```python
from build123d import *

# Parameters (mm, degrees)
SKETCH1_R           = 15
BOSS_EXTRUDE1_DEPTH = 30
SKETCH8_W           = 30
SKETCH8_H           = 15
REVOLVE1_ANGLE      = 180
SKETCH9_W           = 30
SKETCH9_H           = 30
BOSS_EXTRUDE3_DEPTH = 15
SKETCH10_R          = 5
CUT_EXTRUDE1_DEPTH  = 30
SKETCH13_R          = 16
CUT_EXTRUDE2_DEPTH  = 10
SKETCH14_W          = 10
SKETCH14_H          = 15
CUT_EXTRUDE3_DEPTH  = 67
CUT_EXTRUDE4_START  = -7
SKETCH15_R          = 11
SKETCH15_R_2        = 5
CUT_EXTRUDE4_DEPTH  = 7
SKETCH16_R          = 11
SKETCH16_R_2        = 5
CUT_EXTRUDE5_DEPTH  = 7


with BuildPart() as part:
    # Sketch1 → Boss-Extrude1 (new body)
    with BuildSketch(Plane(origin=(0, 0, 0), x_dir=(1, 0, 0), z_dir=(0, 1, 0))):
        with Locations(Location((0, 0, 0), (0, 0, 270))):
            Circle(SKETCH1_R)
    extrude(amount=BOSS_EXTRUDE1_DEPTH)

    # Sketch8 → Revolve1 (revolve)
    with BuildSketch(Plane(origin=(0, 30, 0), x_dir=(1, 0, 0), z_dir=(0, 1, 0))):
        with Locations((0, -7.5)):
            Rectangle(SKETCH8_W, SKETCH8_H)
    revolve(axis=Axis((15, 30, 0), (-1, 0, 0)), revolution_arc=REVOLVE1_ANGLE)

    # Sketch9 → Boss-Extrude3 (add)
    with BuildSketch(Plane.XZ.offset(-30)):
        Rectangle(SKETCH9_W, SKETCH9_H)
    extrude(amount=BOSS_EXTRUDE3_DEPTH)

    # Sketch10 → Cut-Extrude1 (cut)
    with BuildSketch(Plane(origin=(15, 0, 0), x_dir=(0, 0, -1), z_dir=(1, 0, 0))):
        with Locations((0, 30)):
            Circle(SKETCH10_R)
    extrude(amount=-CUT_EXTRUDE1_DEPTH, mode=Mode.SUBTRACT)

    # Sketch13 → Cut-Extrude2 (cut)
    with BuildSketch(Plane(origin=(5, 0, 0), x_dir=(0, 0, -1), z_dir=(1, 0, 0))):
        with Locations((0, 30)):
            Circle(SKETCH13_R)
    extrude(amount=-CUT_EXTRUDE2_DEPTH, mode=Mode.SUBTRACT)

    # Sketch14 → Cut-Extrude3 (cut)
    with BuildSketch(Plane.XY.offset(15)):
        with Locations((0, 22.5)):
            Rectangle(SKETCH14_W, SKETCH14_H)
    extrude(amount=-CUT_EXTRUDE3_DEPTH, mode=Mode.SUBTRACT)

    # Sketch15 → Cut-Extrude4 (cut)
    with BuildSketch(Plane.ZY.offset(15).offset(CUT_EXTRUDE4_START)):
        with Locations((0, 30)):
            Circle(SKETCH15_R)
        with Locations(Location((0, 30, 0), (0, 0, 180))):
            Circle(SKETCH15_R_2, mode=Mode.SUBTRACT)
    extrude(amount=CUT_EXTRUDE4_DEPTH, mode=Mode.SUBTRACT)

    # Sketch16 → Cut-Extrude5 (cut)
    with BuildSketch(Plane(origin=(15, 0, 0), x_dir=(0, 0, -1), z_dir=(1, 0, 0))):
        with Locations(Location((0, 30, 0), (0, 0, 180))):
            Circle(SKETCH16_R)
        with Locations((0, 30)):
            Circle(SKETCH16_R_2, mode=Mode.SUBTRACT)
    extrude(amount=-CUT_EXTRUDE5_DEPTH, mode=Mode.SUBTRACT)


solid = part.part
```
Model file for the job. Use its own axes, mm. A direction names the side the tool comes from. Coordinates: 2 decimals unless noted, no trailing zeros. Order: outer loops, then holes, each group sorted by start corner. A loop starts at its lowest first (then second) coordinate and runs counter-clockwise, first axis right, second up. Notation, with made-up numbers: (-16, 50) - (2, 50) arc R31 ccw to (2, 89) - close; hole circle Ø7 at (52, 44). An arc over 180 degrees is marked (long way). Return JSON: item names as keys, results as strings. Group by question number.
1) Saw through at A-A, the plane y = 21. Write the cut outline in (x, z), plus the area to 3 significant figures.
2) Saw through at C-C, the plane z = 10. Write the cut outline in (x, y).
3) Mould opens along X. For faces 6 (the cylindrical face through (0, 14, 0)), 7 (the cylindrical face through (0.66, 7.395, -14.985)), 8 (the flat face through (8, 35, 2)) say: released by +X, released by -X, zero draft, split by the parting line, or undercut.
4) Saw through at B-B, the plane x = 11.25. Write the cut outline in (y, z), plus the area to 3 significant figures.
5) Probe line 1 (Z direction, x = -5.9, y = 30); line 2 (Z direction, x = 13, y = 30); line 3 (Y direction, x = -5.65, z = 0). List the from-to ranges inside material, lowest first. Write a range as from..to.
6) Flat gauge pins, fed straight in: P1, Ø4, axis at x = 7.5, z = 3, coming from the -Y side; P2, Ø2, axis at x = 5.5, y = 32, coming from the +Z side; P3, Ø8, axis at x = 6, y = 37, coming from the +Z side; P4, Ø17.5, axis at y = 29, z = -1.5, coming from the -X side. Where does each tip first touch, or does it go through?
7) Tool access for faces 1 (the flat face through (12, 15, -11)), 2 (the flat face through (-12, 15, -11)), 3 (the cylindrical face through (-11.45, 19.26, -2.38)), 4 (the flat face through (-12, 15, 12)), 5 (the cylindrical face through (11.55, 40.74, -2.38)): list every direction of +Z, -Z, +X, -X, +Y, -Y with a clear straight run to the whole face (end or side of a thin tool).
8) Saw through at D-D, the plane x = 0. Write the cut outline in (y, z), plus the area to 3 significant figures.
Values found:
{
 "1": {"outline": "(-15, -15) - (-5, -15) - (-5, 15) - (-15, 15) - (-15, 6.32) - (-8, 6.32) - (-8, -6.32) - (-15, -6.32) - close; (5, -15) - (15, -15) - (15, -6.32) - (8, -6.32) - (8, 6.32) - (15, 6.32) - (15, 15) - (5, 15) - close", "area": "423 mm²"},
 "2": {"outline": "(-15, 15) - (-11.18, 15) - (-11.18, 0) - (11.18, 0) - (11.18, 15) - (15, 15) - (15, 25.42) - (8, 25.42) - (8, 34.58) - (15, 34.58) - (15, 41.18) - (5, 41.18) - (5, 15) - (-5, 15) - (-5, 41.18) - (-15, 41.18) - (-15, 34.58) - (-8, 34.58) - (-8, 25.42) - (-15, 25.42) - close"},
 "3": {"face 6": "undercut", "face 7": "split by the parting line", "face 8": "released by +X"},
 "4": {"outline": "(0, -9.92) - (15, -9.92) - (15, -15) - (30, -15) arc R15 ccw to (30, 15) - (15, 15) - (15, 9.92) - (0, 9.92) - close; hole circle Ø22 at (30, 0)", "area": "721 mm²"},
 "5": {"line 1": "z = -15..-5, 5..15", "line 2": "z = -15..-11, 11..15", "line 3": "y = 0..25, 35..45"},
 "6": {"P1": "stops at y = 0", "P2": "stops at z = 14.97", "P3": "stops at z = 14.7", "P4": "stops at x = -8"},
 "7": {"face 1": "-Z, +X, -Y", "face 2": "-Z, -X, -Y", "face 3": "-X", "face 4": "+Z, -X, -Y", "face 5": "+X"},
 "8": {"outline": "(0, -15) - (15, -15) - (15, -5.57) arc R16 cw to (15, 5.57) - (15, 15) - (0, 15) - close", "area": "443 mm²"}
}
